```python
from build123d import *

# Parameters (mm, degrees)
SKETCH1_R           = 2.2
BOSS_EXTRUDE1_DEPTH = 45
SKETCH4_R           = 1.5
CUT_EXTRUDE1_DEPTH  = 51.096706487


with BuildPart() as part:
    # Sketch1 → Boss-Extrude1 (new body)
    with BuildSketch(Plane.XY):
        with Locations(Location((0, 0, 0), (0, 0, 180))):
            Circle(SKETCH1_R)
    extrude(amount=BOSS_EXTRUDE1_DEPTH)

    # Loft1: read off the stored shape, not the designer's step
    # Loft1: loft between two sections, ruled curve by curve
    loft1_from = [
        Edge.make_bspline([(-2.015197815, 0.88259717, 45), (-3.780392156, -3.14779846, 45), (0.250003475, -4.912992801, 45), (2.015197815, -0.88259717, 45), (3.780392156, 3.14779846, 45), (-0.250003475, 4.912992801, 45), (-2.015197815, 0.88259717, 45)], [0, 0, 0, 0, 0.5, 0.5, 0.5, 1, 1, 1, 1], 3, [1, 0.333333333, 0.333333333, 1, 0.333333333, 0.333333333, 1]),
    ]
    loft1_to = [
        Edge.make_bspline([(-1.498749202, -0.061244028, 50), (-1.376261146, -3.058742431, 50), (1.621237257, -2.936254375, 50), (1.498749202, 0.061244028, 50), (1.376261146, 3.058742431, 50), (-1.621237257, 2.936254375, 50), (-1.498749202, -0.061244028, 50)], [0, 0, 0, 0, 0.5, 0.5, 0.5, 1, 1, 1, 1], 3, [1, 0.333333333, 0.333333333, 1, 0.333333333, 0.333333333, 1]),
    ]
    loft1 = Solid(Shell([*[Face.make_surface_from_curves(loft1_from[k], loft1_to[k]) for k in range(1)], Face(Wire(loft1_from)), Face(Wire(loft1_to))]))
    add(loft1)

    # Sketch4 → Cut-Extrude1 (cut, through all)
    with BuildSketch(Plane.XY.offset(50)):
        Circle(SKETCH4_R)
    extrude(amount=-CUT_EXTRUDE1_DEPTH, mode=Mode.SUBTRACT)


solid = part.part
```
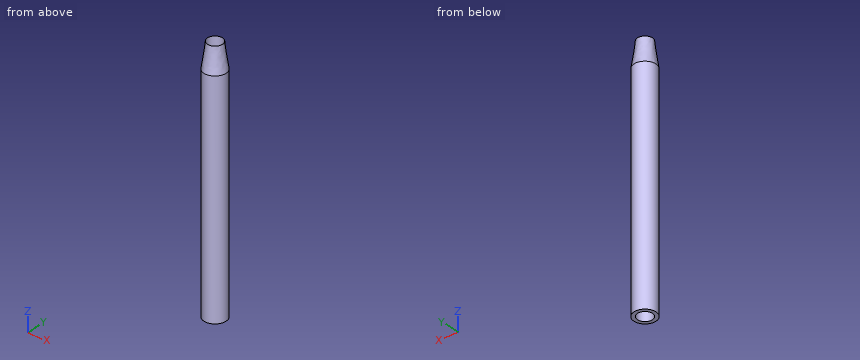
Could you check a few things on this model? Use its own coordinates, in mm. Give positions to 0.01 mm unless a question says otherwise; leave off trailing zeros. Loops run counter-clockwise (first coordinate to the right, second up) from the corner with the lowest first, then second, coordinate; pieces in that order, holes last. Notation, with made-up numbers: (25.5, 61.5) - (62.5, 61.5) arc R33 ccw to (62.5, 98.5) - close; hole circle Ø2 at (33, 1). An arc over 180 degrees is marked (long way). Answer in a Markdown table with one row per item. Add a question column.
Q1. Please list where these lines run through material, in increasing order: L1, parallel to Y at x = 0, z = 11; L2, parallel to Y at x = -0.9, z = 11; L3, parallel to X at y = 0.35, z = 45. Write a range as from..to.
Q2. For pin 1 (1.5 mm diameter, centred on x = 1, z = 5, fed in from +Y); pin 2 (2.5 mm diameter, centred on x = 0, y = 0, fed in from -Z); pin 3 (1 mm diameter, centred on y = -1.5, z = 21, fed in from +X), each with a flat end and sliding along its axis, tell me the tip position at first contact or that it passes through.
Q3. If we section it at A-A (z = 21.5): List the corners of the cut face in (x, y) for me, plus the area to 3 significant figures.
The answers:
| question | item | result |
|---|---|---|
| 1 | L1 | y = -2.2..-1.5, 1.5..2.2 |
| 1 | L2 | y = -2.01..-1.2, 1.2..2.01 |
| 1 | L3 | x = -2.17..-1.46, 1.46..2.17 |
| 2 | pin 1 | stops at y = 2.19 |
| 2 | pin 2 | passes through |
| 2 | pin 3 | stops at x = 1.96 |
| 3 | outline | circle Ø4.4 at (0, 0); hole circle Ø3 at (0, 0) |
| 3 | area | 8.14 mm^2 |
